Could you check a few things on this model? Use its own coordinates, in mm. Face numbers are marked on the shaded views. Round coordinates to 2 decimals unless told otherwise and drop trailing zeros. Write each loop counter-clockwise with the first axis right and the second up, starting at its lowest first coordinate (ties: lowest second). Pieces come first, ordered by that corner, then holes. Notation, with made-up numbers: (58, -34.5) -> (115, -34.5) arc R15 ccw to (115, -21.5) -> close; hole circle Ø9 at (74, -33). An arc over 180 degrees is marked (long way). One line per question, with ' | ' between items. Start each with the question number.
1. Imagine slicing it at B-B, the plane z = 0. List the corners of the cut face in (x, y) for me, and give its area (3 significant figures).
2. Thinking about a two-plate mould opening in Z: for the marked faces 1, 2 and 3, which applies, released by +Z, released by -Z, zero draft, split by the parting line, or undercut?
3. For pin 1 Ø6 at (x, z) = (-10.5, -2.5) entering from +Y; pin 2 Ø5 at (x, z) = (0, 0) entering from +Y; pin 3 Ø5 at (x, z) = (-34, 2) entering from -Y; pin 4 Ø5 at (x, y) = (0, 0) entering from -Z, each with a flat end and sliding along its axis, tell me the tip position at first contact or that it passes through.
4. Imagine slicing it at C-C, the plane z = 4.75. List the corners of the cut face in (x, y) for me, and give its area (3 significant figures).
5. If I drill on line 1 along X through (y, z) = (0, -2.5); line 2 along Z through (x, y) = (0, 22); line 3 along X through (y, z) = (27, 0), over which ranges is the centre line in solid material (lowest first)? Write a range as [from, to].
6. Imagine slicing it at A-A, the plane x = 0. List the corners of the cut face in (y, z) for me.
Solid Edge part; units mm, degrees
sketch "Sketch1" plane through (0, 0, 0) normal (0, -1, 0) x (1, 0, 0)
  line L0 (1.5, -7) -> (46.5, -7)
  line L1 (46.5, -7) -> (42.5, -3.6)
  line L2 (42.5, -3.6) -> (42.5, 3.6)
  line L3 (42.5, 3.6) -> (46.5, 7)
  line L4 (46.5, 7) -> (1.5, 7)
  line L5 (1.5, 7) -> (1.5, -7)
  dimension "D1" = 42.5
revolve "RevolvedProtrusion1" add sketch "Sketch1" angle 360 about axis through (0, 0, 54) along (0, 0, -1)
fillet "Round1" [suppressed]
sketch "Sketch2" plane through (0, 0, 0) normal (0, -1, 0) x (1, 0, 0)
  circle A0 centre (0, 0) radius 1.95
extrude "Ausschnitt_1" cut sketch "Sketch2" against normal blind 55
extrude "Ausschnitt_2" [suppressed]
extrude "HALF" [suppressed]
sketch "Sketch3" plane through (0, 15, 0) normal (0, -1, 0) x (1, 0, 0)
  circle A0 centre (0, 0) radius 3
extrude "Ausschnitt_4" cut sketch "Sketch3" against normal blind 223
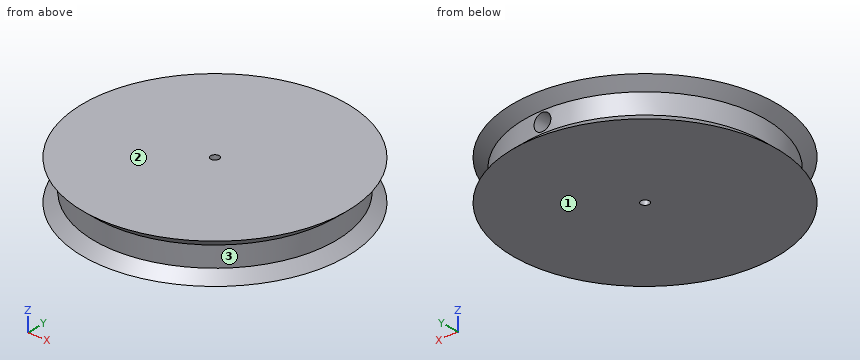
Geometry results:
1) outline: (-3, 15) -> (-3, 42.39) arc R42.5 ccw (long way) to (3, 42.39) -> (3, 15) -> (1.95, 15) -> (1.95, 0) -> (1.5, 0) arc R1.5 cw to (-1.5, 0) -> (-1.95, 0) -> (-1.95, 15) -> close | area: 5,450 mm2
2) face 1: released by -Z | face 2: released by +Z | face 3: undercut
3) pin 1: stops at y = 43.55 | pin 2: stops at y = 15 | pin 3: stops at y = -28.53 | pin 4: stops at z = -7
4) outline: circle Ø87.71 at (0, 0); hole circle Ø3 at (0, 0) | area: 6,030 mm2
5) line 1: x = [-42.5, -1.5], [1.5, 42.5] | line 2: z = [-7, -3], [3, 7] | line 3: x = [-32.82, -3], [3, 32.82]
6) outline: (-46.5, -7) -> (-1.5, -7) -> (-1.5, 7) -> (-46.5, 7) -> (-42.5, 3.6) -> (-42.5, -3.6) -> close; (1.5, -7) -> (46.5, -7) -> (42.5, -3.6) -> (42.5, -3) -> (15, -3) -> (15, -1.95) -> (1.5, -1.95) -> close; (1.5, 1.95) -> (15, 1.95) -> (15, 3) -> (42.5, 3) -> (42.5, 3.6) -> (46.5, 7) -> (1.5, 7) -> close
